Autodesk Fusion 360 part; units mm, degrees
sketch "Esquisse1" plane through (0, 0, 0) normal (0, 0, 1) x (1, 0, 0)
  line L0 (0, 0) -> (200, 0)
  line L1 (200, 0) -> (200, 200)
  line L2 (200, 200) -> (0, 200)
  line L3 (0, 200) -> (0, 0)
  dimension "d18" = 200
  dimension "d19" = 200
extrude "Extrusion1" add sketch "Esquisse1" along normal blind 4
chamfer "Chanfrein1" distance 4 angle 45 1 faces at (66.6667, 133.3333, 0)
sketch "Esquisse2" plane through (0, 0, 4) normal (0, 0, 1) x (-1, 0, 0)
  circle A0 centre (-20, -180) radius 1.5
  circle A1 centre (-180, -180) radius 1.5
  circle A2 centre (-180, -20) radius 1.5
  circle A3 centre (-20, -20) radius 1.5
  line L0 (0, 0) -> (-20, -20)
  line L1 (-200, 0) -> (-180, -20)
  line L2 (-200, 0) -> (-297.1716, 0) construction
  line L3 (0, -200) -> (-20, -180)
  line L4 (-200, -200) -> (-180, -180)
  line L5 (-200, -200) -> (-297.1716, -200) construction
  line L6 (0, -200) -> (0, 0)
  line L7 (0, 0) -> (-200, 0)
  line L8 (-200, 0) -> (-200, -200)
  line L9 (-200, -200) -> (0, -200)
  dimension "d10" = 3
  dimension "d11" = 3
  dimension "d12" = 3
  dimension "d13" = 3
  dimension "d20" = 28.2843
  dimension "d22" = 45
  dimension "d23" = 28.2843
  dimension "d24" = 28.2843
  dimension "d25" = 28.2843
  dimension "d26" = 45
extrude "Extrusion2" cut sketch "Esquisse2" against normal blind 14 contours A0 | A3 | A2 | A1
thread "Filetage1" thread offset 0 thread length 10
thread "Filetage2" thread offset 0 thread length 10
thread "Filetage3" thread offset 0 thread length 10
thread "Filetage4" thread offset 0 thread length 10
equation "d20 = ( sqrt(800) ) * 1 mm"
equation "d23 = ( sqrt(800) ) * 1 mm"
equation "d24 = ( sqrt(800) ) * 1 mm"
equation "d25 = ( sqrt(800) ) * 1 mm"
Can you work these out from the model? Positions are in its coordinate system, mm. Give positions to 0.01 mm unless a question says otherwise; leave off trailing zeros. Order: outer loops, then holes, each group sorted by start corner. A loop starts at its lowest first (then second) coordinate and runs counter-clockwise, first axis right, second up. Notation, with made-up numbers: M -33,48.5 L -17,48.5 A18 ccw -17,77.5 Z; hole C 76,47.5 d9. An arc over 180 degrees is marked long. Use one line per item in the form item = value. Start each with the question number.
Item 1: If I drill on line 1 along X through (y, z) = (180, 1.25); line 2 along Y through (x, z) = (20, 2.75); line 3 along X through (y, z) = (20, 1.75), over which ranges is the centre line in solid material (lowest first)?
Item 2: Will these pins go through, and if not, where does the flat tip stop? pin 1 Ø2 at (x, z) = (99.5, 0.5) entering from +Y; pin 2 Ø2 at (y, z) = (133.5, 1) entering from -X; pin 3 Ø1.5 at (y, z) = (83.5, 2) entering from -X.
Item 3: If we section it at B-B (z = 2.75): Write out the boundary of the cut face in (x, y), then the cut area to 3 significant figures.
Outcome:
q1.line_1 = 2.75 to 18.5, 21.5 to 178.5, 181.5 to 197.25
q1.line_2 = 1.25 to 18.5, 21.5 to 178.5, 181.5 to 198.75
q1.line_3 = 2.25 to 18.5, 21.5 to 178.5, 181.5 to 197.75
q2.pin_1 = 197.5
q2.pin_2 = 2
q2.pin_3 = 1.25
q3.outline = M 1.25,1.25 L 198.75,1.25 L 198.75,198.75 L 1.25,198.75 Z; hole C 20,20 d3; hole C 20,180 d3; hole C 180,20 d3; hole C 180,180 d3
q3.area = 39,000 mm2
